Here's how the part is built. I have some questions about the finished solid (model axes, mm). Face numbers are marked on the shaded views. A direction names the side the tool comes from. Coordinates: 2 decimals unless noted, no trailing zeros. Order: outer loops, then holes, each group sorted by start corner. A loop starts at its lowest first (then second) coordinate and runs counter-clockwise, first axis right, second up. Notation, with made-up numbers: M -30.5,-23 L -23.5,-23 A6 cw -23.5,-17 Z; hole C 84,3.5 d6. An arc over 180 degrees is marked long. Answer as CSV lines item,"result". Start each with the question number.
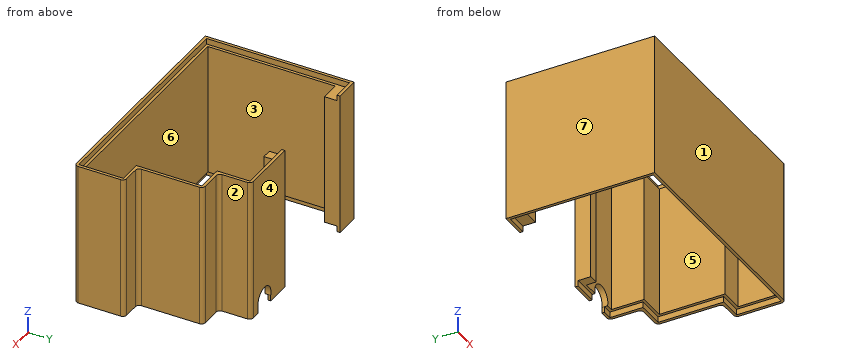
Autodesk Inventor part; units mm, degrees
ref_plane "YZ Plane" through (0, 0, 0) normal (1, 0, 0) x (0, 1, 0)
ref_plane "XZ Plane" through (0, 0, 0) normal (0, 1, 0) x (-1, 0, 0)
ref_plane "XY Plane" through (0, 0, 0) normal (0, 0, 1) x (1, 0, 0)
sketch "Skizze1" plane through (0, 0, 0) normal (0, 0, 1) x (1, 0, 0)
  line L0 (-57.5, 0) -> (57.5, 0)
  line L1 (57.5, 0) -> (57.5, 20)
  line L2 (57.5, 20) -> (45.5, 20)
  line L3 (45.5, 20) -> (45.5, 54)
  line L4 (-57.5, 41) -> (-57.5, 0)
  line L5 (-57.5, 41) -> (-57.5, 41)
  line L6 (-57.5, 54) -> (-57.5, 54)
  line L7 (-57.5, 54) -> (-57.5, 41)
  line L8 (31.5, 71) -> (31.5, 54)
  line L9 (31.5, 54) -> (45.5, 54)
  circle A0 centre (-52, 2.832) radius 1.25
  circle A1 centre (30.6262, 2.832) radius 1.25
  circle A2 centre (30.6262, 51.168) radius 1.25
  circle A3 centre (-44.507, 51.168) radius 1.25
  line L10 (33.3762, 2.832) -> (33.3762, 0)
  line L11 (33.3762, 0) -> (27.8762, 0)
  line L12 (27.8762, 0) -> (27.8762, 2.832)
  arc A4 (33.3762, 2.832) -> (27.8762, 2.832) centre (30.6262, 2.832) ccw
  line L13 (-49.25, 0) -> (-49.25, 2.832)
  line L14 (-54.75, 0) -> (-54.75, 2.832)
  line L15 (-49.25, 0) -> (-54.75, 0)
  arc A5 (-49.25, 2.832) -> (-54.75, 2.832) centre (-52, 2.832) ccw
  line L16 (33.3762, 51.168) -> (33.3762, 54)
  line L17 (33.3762, 54) -> (27.8762, 54)
  line L18 (27.8762, 54) -> (27.8762, 51.168)
  arc A6 (27.8762, 51.168) -> (33.3762, 51.168) centre (30.6262, 51.168) ccw
  line L19 (-41.757, 51.168) -> (-41.757, 54)
  line L20 (-41.757, 54) -> (-47.257, 54)
  line L21 (-47.257, 54) -> (-47.257, 51.168)
  arc A7 (-47.257, 51.168) -> (-41.757, 51.168) centre (-44.507, 51.168) ccw
  line L22 (-57.5, 54) -> (31.5, 54)
  line L23 (31.5, 54) -> (31.5, 57)
  line L24 (31.5, 57) -> (-57.5, 57)
  line L25 (-57.5, 57) -> (-57.5, 54)
  line L26 (31.5, 71) -> (-57.5, 71)
  line L27 (-57.5, 71) -> (-57.5, 54)
  line L28 (48.5, 23) -> (60.5, 23)
  line L29 (60.5, 23) -> (60.5, -3)
  line L30 (60.5, -3) -> (-60.5, -3)
  line L31 (-60.5, -3) -> (-60.5, 44)
  line L32 (-60.5, 44) -> (-60.5, 44)
  line L33 (-60.5, 44) -> (-60.5, 57)
  line L34 (-60.5, 57) -> (-60.5, 57)
  line L35 (-60.5, 57) -> (-60.5, 74)
  line L36 (-60.5, 74) -> (34.5, 74)
  line L37 (34.5, 74) -> (34.5, 57)
  line L38 (34.5, 57) -> (48.5, 57)
  line L39 (48.5, 57) -> (48.5, 23)
  line L40 (-57.5, 71) -> (-47.5, 71)
  line L41 (-47.5, 71) -> (-47.5, 66)
  line L42 (-47.5, 66) -> (-57.5, 66)
  line L43 (-57.5, 66) -> (-57.5, 71)
  line L44 (8.5, 71) -> (3.5, 71)
  line L45 (3.5, 71) -> (3.5, 66)
  line L46 (3.5, 66) -> (8.5, 66)
  line L47 (8.5, 66) -> (8.5, 71)
  line L48 (-47.5, 71) -> (3.5, 71)
  line L49 (3.5, 71) -> (3.5, 74)
  line L50 (3.5, 74) -> (-47.5, 74)
  line L51 (-47.5, 74) -> (-47.5, 71)
  point P0 (0, 0)
  point P1 (0, 0)
  point P2 (0, 0)
  point P3 (0, 0)
  dimension "d0" = 115
  dimension "d1" = 12
  dimension "d2" = 20
  dimension "d3" = 41
  dimension "d4" = 54
  dimension "d5" = 5.5
  dimension "d6" = 82.6262
  dimension "d7" = 2.5
  dimension "d8" = 2.832
  dimension "d9" = 7.493
  dimension "d10" = 48.336
  dimension "d11" = 5.5
  dimension "d12" = 5.5
  dimension "d13" = 5.5
  dimension "d14" = 5.5
  dimension "d15" = 3
  dimension "d16" = 0
  dimension "d17" = 89
  dimension "d18" = 71
  dimension "d19" = 3
  dimension "d20" = 2.832
  dimension "d29" = 10
  dimension "d30" = 5
  dimension "d31" = 5
  dimension "d34" = 51
  dimension "d40" = 0
extrude "Extrusion1" add sketch "Skizze1" along normal blind 68 contours L0 L1 L2 L3 L9 L8 L26 L49 L36 L37 L38 L39 L28 L29 L30 L31 L33 L35 L51 L27 L25 L7 L4 | L27 L26 L41 L42 | L47 L46 L45 L26
sketch "Skizze3" plane through (3.5, 74, 0) normal (0, 1, 0) x (1, 0, 0)
  line L0 (31, 0) -> (31, -68)
  line L1 (28, 0) -> (5, 0)
  arc A0 (13, 0) -> (24.5, 0) centre (18.75, -1.7139) ccw
  line L2 (13, 0) -> (24.5, 0)
  point P0 (-3.5, 0)
  dimension "d35" = 6
  dimension "d36" = 12.25
  dimension "d39" = 11.5
extrude "Extrusion4" cut sketch "Skizze3" against normal up to surface (3 mm away)
sketch "Skizze4" plane through (0, 0, 68) normal (0, 0, 1) x (1, 0, 0)
  line L0 (57.5, 0) -> (-57.5, 0)
  line L1 (-47.5, 74) -> (-60.5, 74)
  line L2 (-60.5, 74) -> (-60.5, -3)
  line L3 (48.5, 23) -> (48.5, 57)
  line L4 (48.5, 57) -> (34.5, 57)
  line L5 (34.5, 74) -> (3.5, 74)
  line L6 (-47.5, 74) -> (-60.5, 74)
  line L7 (-60.5, 74) -> (-60.5, -3)
  line L8 (-60.5, -3) -> (60.5, -3)
  line L9 (60.5, -3) -> (60.5, 23)
  line L10 (60.5, 23) -> (48.5, 23)
  line L11 (48.5, 23) -> (48.5, 57)
  line L12 (48.5, 57) -> (34.5, 57)
  line L13 (34.5, 57) -> (34.5, 74)
  line L14 (34.5, 74) -> (3.5, 74)
  line L15 (3.5, 72.5) -> (33, 72.5)
  line L16 (33, 72.5) -> (33, 55.5)
  line L17 (33, 55.5) -> (47, 55.5)
  line L18 (47, 55.5) -> (47, 21.5)
  line L19 (47, 21.5) -> (59, 21.5)
  line L20 (59, 21.5) -> (59, -1.5)
  line L21 (59, -1.5) -> (-59, -1.5)
  line L22 (-59, -1.5) -> (-59, 72.5)
  line L23 (-59, 72.5) -> (-47.5, 72.5)
  line L24 (3.5, 72.5) -> (3.5, 74)
  line L25 (-47.5, 72.5) -> (-47.5, 74)
  point P0 (0, 0)
  dimension "d41" = 1.5
extrude "Extrusion5" add sketch "Skizze4" along normal blind 3
sketch "Skizze5" plane through (0, 0, 0) normal (0, 0, -1) x (-1, 0, 0)
  line L0 (-34.5, 74) -> (-34.5, 57)
  line L1 (-48.5, 23) -> (-60.5, 23)
  line L2 (47.5, 74) -> (47.5, 66)
  line L3 (-28, 74) -> (-34.5, 74)
  line L4 (-34.5, 74) -> (-34.5, 57)
  line L5 (-34.5, 57) -> (-48.5, 57)
  line L6 (-48.5, 57) -> (-48.5, 23)
  line L7 (-48.5, 23) -> (-60.5, 23)
  line L8 (-60.5, 23) -> (-60.5, -3)
  line L9 (60.5, 74) -> (60.5, -3)
  line L10 (-60.5, -3) -> (60.5, -3)
  line L11 (60.5, -3) -> (60.5, 74)
  line L12 (60.5, 74) -> (47.5, 74)
  line L13 (-28, 72.5) -> (-33, 72.5)
  line L14 (-33, 72.5) -> (-33, 55.5)
  line L15 (-33, 55.5) -> (-47, 55.5)
  line L16 (-47, 55.5) -> (-47, 21.5)
  line L17 (-47, 21.5) -> (-59, 21.5)
  line L18 (-59, 21.5) -> (-59, -1.5)
  line L19 (-59, -1.5) -> (59, -1.5)
  line L20 (59, -1.5) -> (59, 72.5)
  line L21 (59, 72.5) -> (47.5, 72.5)
  line L22 (-28, 74) -> (-28, 72.5)
  line L23 (47.5, 74) -> (60.5, 74)
  line L24 (47.5, 66) -> (47.5, 72.5)
  line L25 (47.5, 74) -> (47.5, 72.5)
  line L26 (-3.5, 74) -> (-16.5, 74)
  line L27 (-3.5, 72.5) -> (-3.5, 66)
  line L28 (-16.5, 74) -> (-3.5, 74)
  line L29 (-3.5, 74) -> (-3.5, 72.5)
  line L30 (-3.5, 72.5) -> (-16.5, 72.5)
  line L31 (-16.5, 72.5) -> (-16.5, 74)
  point P0 (0, 0)
  dimension "d44" = 1.5
  dimension "d47" = 1.5
extrude "Extrusion6" add sketch "Skizze5" along normal blind 3
fillet "Rundung1" radius 2 6 edges at (60.5, -3, 34) (60.5, 23, 34) (48.5, 57, 34) (34.5, 74, 34) (34.5, 57, 34) (48.5, 23, 34)
equation "\"d47\" = d44"
properties part number "Display"
1) Will these pins go through, and if not, where does the flat tip stop? pin 1 Ø1.6 at (y, z) = (73.5, -1.5) entering from +X; pin 2 Ø7 at (x, z) = (22.25, 1.71) entering from +Y; pin 3 Ø12 at (y, z) = (54.5, 59.5) entering from +X.
2) I need wall thicknesses on line 1 (X direction, y = 69, z = 23.5); line 2 (X direction, y = 43, z = 27); line 3 (X direction, y = 16, z = 49). Which ranges of each line are inside material? Lowest first, please. Write a range as [from, to].
3) Suppose I cut it at C-C on x = -5. Please give me the cut outline in (y, z).
4) If we mould it in two halves opening along Y, with no side actions, what happens to the marked faces 4, 5, 6 and 7? For each: released by +Y, released by -Y, zero draft, split by the parting line, or undercut.
5) Suppose I cut it at D-D on z = 61. Please give me the cut outline in (x, y), plus the area to 3 significant figures.
6) Suppose I cut it at A-A on x = 39. Please give me the cut outline in (y, z).
7) Which directions (+Z, -Z, +X, -X, +Y, -Y) give clear straight access to the entire face, cutting with the end or side of a thin tool? Please do the marked faces 1, 2 and 3.
8) Suppose I cut it at B-B on y = 27.5. Please give me the cut outline in (x, z), plus the area to 3 significant figures.
Output:
1,pin 1,"x = 34.37"
1,pin 2,"y = 0"
1,pin 3,"x = 48.5"
2,line 1,"[-60.5, -47.5], [3.5, 8.5], [31.5, 34.5]"
2,line 2,"[-60.5, -57.5], [45.5, 48.5]"
2,line 3,"[-60.5, -57.5], [57.5, 60.5]"
3,outline,"M -3,-3 L -1.5,-3 L -1.5,0 L 0,0 L 0,68 L -1.5,68 L -1.5,71 L -3,71 Z"
4,face 4,"released by +Y"
4,face 5,"undercut"
4,face 6,"undercut"
4,face 7,"zero draft"
5,outline,"M -60.5,-3 L 58.5,-3 A2 ccw 60.5,-1 L 60.5,21 A2 ccw 58.5,23 L 50.5,23 A2 cw 48.5,25 L 48.5,55 A2 ccw 46.5,57 L 36.5,57 A2 cw 34.5,59 L 34.5,72 A2 ccw 32.5,74 L 3.5,74 L 3.5,66 L 8.5,66 L 8.5,71 L 31.5,71 L 31.5,54 L 45.5,54 L 45.5,20 L 57.5,20 L 57.5,0 L -57.5,0 L -57.5,66 L -47.5,66 L -47.5,74 L -60.5,74 Z"
5,area,"1,070 mm²"
6,outline,"M -3,-3 L -1.5,-3 L -1.5,0 L 0,0 L 0,68 L -1.5,68 L -1.5,71 L -3,71 Z; M 54,0 L 55.5,0 L 55.5,-3 L 57,-3 L 57,71 L 55.5,71 L 55.5,68 L 54,68 Z"
7,face 1,"+Z, -Z, +X, -X, -Y"
7,face 2,"+Z, -Z, +X, +Y"
7,face 3,"+Z, -Z"
8,outline,"M -60.5,-3 L -59,-3 L -59,0 L -57.5,0 L -57.5,68 L -59,68 L -59,71 L -60.5,71 Z; M 45.5,0 L 47,0 L 47,-3 L 48.5,-3 L 48.5,71 L 47,71 L 47,68 L 45.5,68 Z"
8,area,"426 mm²"
